Autodesk Inventor part; units mm, degrees
ref_plane "YZ Plane" through (0, 0, 0) normal (1, 0, 0) x (0, 1, 0)
ref_plane "XZ Plane" through (0, 0, 0) normal (0, 1, 0) x (-1, 0, 0)
ref_plane "XY Plane" through (0, 0, 0) normal (0, 0, 1) x (1, 0, 0)
sketch "Szkic1" plane through (0, 0, 0) normal (0, 0, 1) x (1, 0, 0)
  line L0 (0, 0) -> (70, 0) construction
  line L1 (70, 0) -> (70, 70) construction
  line L2 (70, 70) -> (0, 70) construction
  line L3 (0, 70) -> (0, 0) construction
  line L4 (0, 0) -> (6, 0) construction
  line L5 (6, 0) -> (6, 70) construction
  line L6 (6, 70) -> (0, 70) construction
  line L7 (0, 70) -> (0, 0) construction
  line L8 (0, 0) -> (70, 0) construction
  line L9 (70, 0) -> (70, 6) construction
  line L10 (70, 6) -> (0, 6) construction
  line L11 (0, 6) -> (0, 0) construction
  line L12 (6, 6) -> (174, 6) construction
  line L13 (174, 6) -> (174, 174) construction
  line L14 (174, 174) -> (6, 174) construction
  line L15 (6, 174) -> (6, 6) construction
  line L16 (90, 174) -> (90, 6) construction
  circle A0 centre (90, 90) radius 65 construction
  line L17 (0, 0) -> (70, 0)
  line L18 (0, 0) -> (0, 70)
  line L19 (0, 70) -> (28.1534, 70)
  line L20 (70, 0) -> (70, 28.1534)
  arc A1 (28.1534, 70) -> (70, 28.1534) centre (90, 90) ccw
  dimension "d23" = 70
  dimension "d24" = 70
  dimension "d25" = 6
  dimension "d26" = 6
  dimension "d27" = 168
  dimension "d28" = 168
  dimension "d29" = 130
extrude "Wyciągnięcie proste1" add sketch "Szkic1" along normal blind 6
equation "\"d23\" = d24"
properties part number "Naroznik_60x60"
Source: CAD feature listing. Evaluate the final solid. Frame: model axes, mm. Round coordinates to 2 decimals unless told otherwise and drop trailing zeros. Loops run counter-clockwise (first coordinate to the right, second up) from the corner with the lowest first, then second, coordinate; pieces in that order, holes last. Notation, with made-up numbers: M -8.75,44 L 6.25,44 A23 cw 6.25,81 Z; hole C 32.5,-26.75 d2. An arc over 180 degrees is marked long. Return JSON: item names as keys, results as strings. Group by question number.
1. Section query C-C on y = 46.5. Output: boundary loops of the cut face in (x, z).
2. Section query A-A on z = 1.6. Output: boundary loops of the cut face in (x, y), and give its area (3 significant figures).
3. Material intervals for line 1 along Y through (x, z) = (64.5, 1.3); line 2 along Y through (x, z) = (33, 0.9); line 3 along X through (y, z) = (39, 2.1), sorted ascending. Write a range as from..to.
4. Pin query (flat end, axial travel): pin 1 (1 mm diameter, centred on x = 37, z = 1, fed in from +Y). Return the tip coordinate at first contact, or that it passes through.
5. Section query B-B on x = 65.5. Output: boundary loops of the cut face in (y, z).
Checks:
{
 "1": {"outline": "M 0,0 L 41.7,0 L 41.7,6 L 0,6 Z"},
 "2": {"outline": "M 0,0 L 70,0 L 70,28.15 A65 cw 28.15,70 L 0,70 Z", "area": "3,740 mm²"},
 "3": {"line 1": "y = 0..30.21", "line 2": "y = 0..58.76", "line 3": "x = 0..49.7"},
 "4": {"pin 1": "stops at y = 53.08"},
 "5": {"outline": "M 0,0 L 29.79,0 L 29.79,6 L 0,6 Z"}
}
